Geometry: final body of the model. Coordinates: model frame, mm. Coordinates: 2 decimals unless noted, no trailing zeros. Loops run counter-clockwise (first coordinate to the right, second up) from the corner with the lowest first, then second, coordinate; pieces in that order, holes last. Notation, with made-up numbers: (81.5, -39.75) -> (100.5, -39.75) arc R18 cw to (100.5, -27.75) -> close; hole circle Ø3 at (-39.5, 73). An arc over 180 degrees is marked (long way). One line per item, written item: value. Start each with the question number.
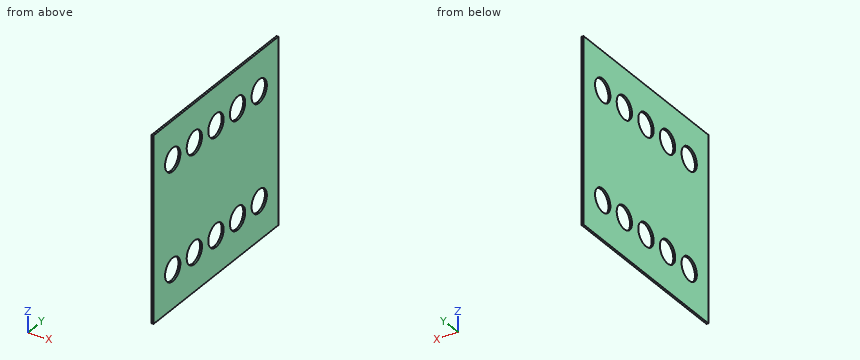
from build123d import *

# Parameters (mm, degrees)
PAD_DEPTH    = 5
SKETCH002_R  = 30
POCKET_DEPTH = 5.001


with BuildPart() as part:
    # Sketch → Pad (new body)
    with BuildSketch(Plane.YZ):
        Polygon((0, 0), (0, 480), (490, 480), (490, 0), (245, 0), align=None)
    extrude(amount=-PAD_DEPTH)

    # Sketch002 (on Face6 of Pad) → Pocket (cut, through all)
    with BuildSketch(Plane.YZ):
        with Locations((245, 380)):
            Circle(SKETCH002_R)
        with Locations((245, 100)):
            Circle(SKETCH002_R)
        with Locations((75.312646, 380)):
            Circle(SKETCH002_R)
        with Locations((75.312646, 100)):
            Circle(SKETCH002_R)
        with Locations((160.156323, 100)):
            Circle(SKETCH002_R)
        with Locations((329.843677, 100)):
            Circle(SKETCH002_R)
        with Locations((414.687354, 100)):
            Circle(SKETCH002_R)
        with Locations((414.687354, 380)):
            Circle(SKETCH002_R)
        with Locations((329.843677, 380)):
            Circle(SKETCH002_R)
        with Locations((160.156323, 380)):
            Circle(SKETCH002_R)
    extrude(amount=-POCKET_DEPTH, mode=Mode.SUBTRACT)


solid = part.part
1. Section C-C on y = 245. Return the cut outline in (x, z), plus the area to 3 significant figures.
2. Section A-A on z = 100. Return the cut outline in (x, y).
3. Section B-B on x = -4.05. Count the separate pieces of the cut face and the enclosed holes in it, plus the area to 3 significant figures.
4. Line query: L1, parallel to Z at x = -1.35, y = 245; L2, parallel to Y at x = -0.3, z = 357; L3, parallel to Z at x = -2.5, y = 149.5. Output: solid intervals per line, ascending. Write a range as [from, to].
Checks:
1. outline: (-5, 0) -> (0, 0) -> (0, 70) -> (-5, 70) -> close; (-5, 130) -> (0, 130) -> (0, 350) -> (-5, 350) -> close; (-5, 410) -> (0, 410) -> (0, 480) -> (-5, 480) -> close
1. area: 1,800 mm²
2. outline: (-5, 0) -> (0, 0) -> (0, 45.31) -> (-5, 45.31) -> close; (-5, 105.31) -> (0, 105.31) -> (0, 130.16) -> (-5, 130.16) -> close; (-5, 190.16) -> (0, 190.16) -> (0, 215) -> (-5, 215) -> close; (-5, 275) -> (0, 275) -> (0, 299.84) -> (-5, 299.84) -> close; (-5, 359.84) -> (0, 359.84) -> (0, 384.69) -> (-5, 384.69) -> close; (-5, 444.69) -> (0, 444.69) -> (0, 490) -> (-5, 490) -> close
3. separate pieces: 1
3. enclosed holes: 10
3. area: 207,000 mm²
4. L1: [0, 70], [130, 350], [410, 480]
4. L2: [0, 56.05], [94.57, 140.89], [179.42, 225.74], [264.26, 310.58], [349.11, 395.43], [433.95, 490]
4. L3: [0, 71.96], [128.04, 351.96], [408.04, 480]
